Geometry check sheet. Reference: the model listing, model coordinates, mm. Face numbers are marked on the shaded views. A direction names the side the tool comes from. Give positions to 0.01 mm unless a question says otherwise; leave off trailing zeros. Loops run counter-clockwise (first coordinate to the right, second up) from the corner with the lowest first, then second, coordinate; pieces in that order, holes last. Notation, with made-up numbers: (-15.5, 73.5) - (1.5, 73.5) arc R20 ccw to (1.5, 103.5) - close; hole circle Ø10 at (-26.75, 29). An arc over 180 degrees is marked (long way). Use a Markdown table: item, result. Add a question column.
1. Depth check by flat-ended pin: P1, Ø4.5, axis at x = 20, z = 20, coming from the +Y side. Enter the tip coordinate at first touch or a pass-through.
2. Material ranges on L1, parallel to X at y = 4.5, z = 20; L2, parallel to X at y = 2, z = -20 (3 decimals), recorded low to high.
3. Cross-section at C-C on x = 0. Enter the section's corners in (y, z) (3 decimals).
4. Cross-section at B-B on y = 1.5. Enter the section's corners in (x, z) (3 decimals), and give its area (3 significant figures).
5. Draft check along X on the marked faces 1, 2 and 3. Enter one of: pulls with the +X half, pulls with the -X half, needs draft (parallel to the pull), parting line crosses it, or undercut.
6. Cross-section at D-D on y = 7.25. Enter the section's corners in (x, z) (3 decimals), and give its area (3 significant figures).
7. Set-up check for the marked faces 4 and 5: record each of +Z, -Z, +X, -X, +Y, -Y from which the full face is reachable in a straight line by a thin tool's end or side.
8. Cross-section at A-A on z = -1. Enter the section's corners in (x, y) (3 decimals), and give its area (3 significant figures).
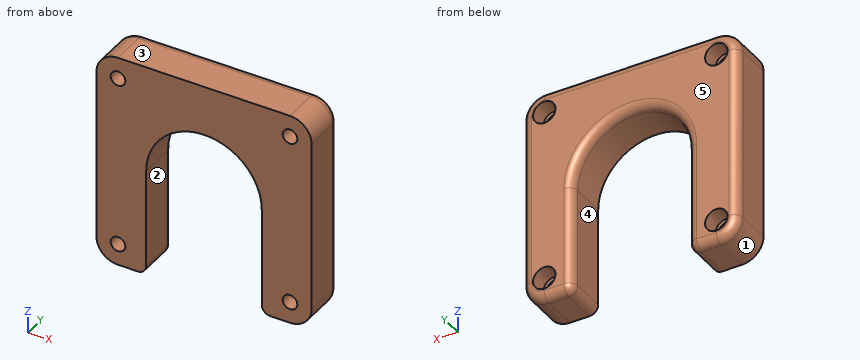
from build123d import *

# Parameters (mm, degrees)
BOSS_EXTRUDE1_DEPTH          = 10
SKETCH1_4_R                  = 1.7
CUT_EXTRUDE1_DEPTH           = 37.742346142
CUT_EXTRUDE2_START           = 10
SKETCH1_5_R                  = 2.6
CUT_EXTRUDE2_DEPTH           = 3.9
CUT_EXTRUDE2_DRAFT           = -1.5
CUT_EXTRUDE2_PROFILE_2_DEPTH = 3.9
CUT_EXTRUDE2_PROFILE_2_DRAFT = -1.5
CUT_EXTRUDE2_PROFILE_3_DEPTH = 3.9
CUT_EXTRUDE2_PROFILE_3_DRAFT = -1.5
CUT_EXTRUDE2_PROFILE_4_DEPTH = 3.9
CUT_EXTRUDE2_PROFILE_4_DRAFT = -1.5
FILLET1_R                    = 2
FILLET2_R                    = 2


with BuildPart() as part:
    # Sketch1 → Boss-Extrude1 (new body)
    with BuildSketch(Plane(origin=(0, 0, 0), x_dir=(1, 0, 0), z_dir=(0, 1, 0))):
        with BuildLine():
            Line((-20, -25), (20, -25))
            ThreePointArc((20, -25), (23.535533906, -23.535533906), (25, -20))
            Line((25, -20), (25, 20))
            ThreePointArc((25, 20), (23.535533906, 23.535533906), (20, 25))
            Line((20, 25), (-20, 25))
            ThreePointArc((-20, 25), (-23.535533906, 23.535533906), (-25, 20))
            Line((-25, 20), (-25, -20))
            ThreePointArc((-25, -20), (-23.535533906, -23.535533906), (-20, -25))
        make_face()
    extrude(amount=BOSS_EXTRUDE1_DEPTH)

    # Sketch1<4> → Cut-Extrude1 (cut, through all)
    with BuildSketch(Plane(origin=(0, 0, 0), x_dir=(1, 0, 0), z_dir=(0, 1, 0))):
        with BuildLine():
            Line((13.435, 25), (-13.435, 25))
            Line((-13.435, 25), (-13.435, 0))
            ThreePointArc((-13.435, 0), (0, -13.435), (13.435, 0))
            Line((13.435, 0), (13.435, 25))
        make_face()
        with Locations(Location((-20, 20, 0), (0, 0, 270))):
            Circle(SKETCH1_4_R)
        with Locations(Location((-20, -20, 0), (0, 0, 90))):
            Circle(SKETCH1_4_R)
        with Locations(Location((20, -20, 0), (0, 0, 90))):
            Circle(SKETCH1_4_R)
        with Locations(Location((20, 20, 0), (0, 0, 270))):
            Circle(SKETCH1_4_R)
    extrude(amount=CUT_EXTRUDE1_DEPTH, mode=Mode.SUBTRACT)


with BuildPart() as cut_extrude2_tool:
    # Sketch1<5> → Cut-Extrude2 (with draft: the straight prism first)
    with BuildSketch(Plane(origin=(0, 0, 0), x_dir=(1, 0, 0), z_dir=(0, 1, 0)).offset(CUT_EXTRUDE2_START)):
        with Locations((-20, 20)):
            Circle(SKETCH1_5_R)
    extrude(amount=-CUT_EXTRUDE2_DEPTH)
    # Cut-Extrude2: the draft: its side faces are tilted about the plane it starts from
    cut_extrude2_sides = [cut_extrude2_tool.faces().sort_by_distance(p)[0] for p in [
        (-22.6, 8.05, -20),
    ]]
    draft(cut_extrude2_sides, Plane(origin=(0, 0, 0), x_dir=(1, 0, 0), z_dir=(0, 1, 0)).offset(CUT_EXTRUDE2_START), CUT_EXTRUDE2_DRAFT)


with BuildPart() as part_1:
    add(part.part)

    # Cut-Extrude2: cut by cut_extrude2_tool
    add(cut_extrude2_tool.part, mode=Mode.SUBTRACT)


with BuildPart() as cut_extrude2_profile_2_tool:
    # Sketch1<5> → Cut-Extrude2 profile 2 (with draft: the straight prism first)
    with BuildSketch(Plane(origin=(0, 0, 0), x_dir=(1, 0, 0), z_dir=(0, 1, 0)).offset(CUT_EXTRUDE2_START)):
        with Locations((20, 20)):
            Circle(SKETCH1_5_R)
    extrude(amount=-CUT_EXTRUDE2_PROFILE_2_DEPTH)
    # Cut-Extrude2 profile 2: the draft: its side faces are tilted about the plane it starts from
    cut_extrude2_profile_2_sides = [cut_extrude2_profile_2_tool.faces().sort_by_distance(p)[0] for p in [
        (17.4, 8.05, -20),
    ]]
    draft(cut_extrude2_profile_2_sides, Plane(origin=(0, 0, 0), x_dir=(1, 0, 0), z_dir=(0, 1, 0)).offset(CUT_EXTRUDE2_START), CUT_EXTRUDE2_PROFILE_2_DRAFT)


with BuildPart() as part_2:
    add(part_1.part)

    # Cut-Extrude2 profile 2: cut by cut_extrude2_profile_2_tool
    add(cut_extrude2_profile_2_tool.part, mode=Mode.SUBTRACT)


with BuildPart() as cut_extrude2_profile_3_tool:
    # Sketch1<5> → Cut-Extrude2 profile 3 (with draft: the straight prism first)
    with BuildSketch(Plane(origin=(0, 0, 0), x_dir=(1, 0, 0), z_dir=(0, 1, 0)).offset(CUT_EXTRUDE2_START)):
        with Locations((-20, -20)):
            Circle(SKETCH1_5_R)
    extrude(amount=-CUT_EXTRUDE2_PROFILE_3_DEPTH)
    # Cut-Extrude2 profile 3: the draft: its side faces are tilted about the plane it starts from
    cut_extrude2_profile_3_sides = [cut_extrude2_profile_3_tool.faces().sort_by_distance(p)[0] for p in [
        (-22.6, 8.05, 20),
    ]]
    draft(cut_extrude2_profile_3_sides, Plane(origin=(0, 0, 0), x_dir=(1, 0, 0), z_dir=(0, 1, 0)).offset(CUT_EXTRUDE2_START), CUT_EXTRUDE2_PROFILE_3_DRAFT)


with BuildPart() as part_3:
    add(part_2.part)

    # Cut-Extrude2 profile 3: cut by cut_extrude2_profile_3_tool
    add(cut_extrude2_profile_3_tool.part, mode=Mode.SUBTRACT)


with BuildPart() as cut_extrude2_profile_4_tool:
    # Sketch1<5> → Cut-Extrude2 profile 4 (with draft: the straight prism first)
    with BuildSketch(Plane(origin=(0, 0, 0), x_dir=(1, 0, 0), z_dir=(0, 1, 0)).offset(CUT_EXTRUDE2_START)):
        with Locations((20, -20)):
            Circle(SKETCH1_5_R)
    extrude(amount=-CUT_EXTRUDE2_PROFILE_4_DEPTH)
    # Cut-Extrude2 profile 4: the draft: its side faces are tilted about the plane it starts from
    cut_extrude2_profile_4_sides = [cut_extrude2_profile_4_tool.faces().sort_by_distance(p)[0] for p in [
        (17.4, 8.05, 20),
    ]]
    draft(cut_extrude2_profile_4_sides, Plane(origin=(0, 0, 0), x_dir=(1, 0, 0), z_dir=(0, 1, 0)).offset(CUT_EXTRUDE2_START), CUT_EXTRUDE2_PROFILE_4_DRAFT)


with BuildPart() as part_4:
    add(part_3.part)

    # Cut-Extrude2 profile 4: cut by cut_extrude2_profile_4_tool
    add(cut_extrude2_profile_4_tool.part, mode=Mode.SUBTRACT)

    # Fillet1
    fillet1_edges = [part_4.edges().sort_by_distance(p)[0] for p in [
        (-13.435, 10, -12.5),
        (-13.435, 5, -25),
        (13.435, 5, -25),
        (0, 10, 13.435),
        (13.435, 10, -12.5),
    ]]
    fillet(fillet1_edges, radius=FILLET1_R)

    # Fillet2
    # the kernel refuses this fillet: 2 mm, written as the material it takes off along each edge
    with BuildSketch(Plane(origin=(15.435, 8, -23), x_dir=(0, 1, 0), z_dir=(0, 0, -1))) as fillet2_piece_1_section:
        Polygon((0, 0), (FILLET2_R, 0), (FILLET2_R, -FILLET2_R), (0, -FILLET2_R), align=None)
    fillet2_piece_1 = extrude(amount=FILLET2_R, mode=Mode.PRIVATE)
    fillet2_piece_1 = fillet2_piece_1 - Plane(origin=(15.435, 8, -23), x_dir=(0.7071067811865475, -0.7071067811865475, 0), z_dir=(0, 0, -1)) * Sphere(FILLET2_R, mode=Mode.PRIVATE)
    add(fillet2_piece_1, mode=Mode.SUBTRACT)
    with BuildSketch(Plane(origin=(-15.435, 8, -23), x_dir=(0, 1, 0), z_dir=(0, 0, -1))) as fillet2_piece_2_section:
        Polygon((0, 0), (FILLET2_R, 0), (FILLET2_R, FILLET2_R), (0, FILLET2_R), align=None)
    fillet2_piece_2 = extrude(amount=FILLET2_R, mode=Mode.PRIVATE)
    fillet2_piece_2 = fillet2_piece_2 - Plane(origin=(-15.435, 8, -23), x_dir=(-0.7071067811865475, -0.7071067811865475, 0), z_dir=(0, 0, -1)) * Sphere(FILLET2_R, mode=Mode.PRIVATE)
    add(fillet2_piece_2, mode=Mode.SUBTRACT)
    with BuildSketch(Plane(origin=(-20, 10, -20), x_dir=(0, 0, -1), z_dir=(1, 0, 0))) as fillet2_piece_3:
        with BuildLine():
            CenterArc((5 - FILLET2_R, -FILLET2_R), FILLET2_R, 0, 90)
            Line((5 - FILLET2_R, 0), (5, 0))
            Line((5, 0), (5, -FILLET2_R))
        make_face()
    revolve(axis=Axis((-20, 10, -20), (0, 1, 0)), revolution_arc=90, mode=Mode.SUBTRACT)
    with BuildSketch(Plane(origin=(-15.435, 10, -25), x_dir=(0, -1, 0), z_dir=(-1, 0, 0)), Plane(origin=(20, 10, -25), x_dir=(0, -1, 0), z_dir=(-1, 0, 0))) as fillet2_piece_4:
        with BuildLine():
            CenterArc((FILLET2_R, FILLET2_R), FILLET2_R, 180, 90)
            Line((0, FILLET2_R), (0, 0))
            Line((0, 0), (FILLET2_R, 0))
        make_face()
    extrude(amount=4.565, mode=Mode.SUBTRACT)
    with BuildSketch(Plane(origin=(20, 10, -20), x_dir=(1, 0, 0), z_dir=(0, 0, 1))) as fillet2_piece_5:
        with BuildLine():
            CenterArc((5 - FILLET2_R, -FILLET2_R), FILLET2_R, 0, 90)
            Line((5 - FILLET2_R, 0), (5, 0))
            Line((5, 0), (5, -FILLET2_R))
        make_face()
    revolve(axis=Axis((20, 10, -20), (0, 1, 0)), revolution_arc=90, mode=Mode.SUBTRACT)
    with BuildSketch(Plane(origin=(25, 10, 20), x_dir=(0, -1, 0), z_dir=(0, 0, -1)), Plane(origin=(-20, 10, 25), x_dir=(0, -1, 0), z_dir=(1, 0, 0)), Plane(origin=(-25, 10, -20), x_dir=(0, -1, 0), z_dir=(0, 0, 1))) as fillet2_piece_6:
        with BuildLine():
            CenterArc((FILLET2_R, FILLET2_R), FILLET2_R, 180, 90)
            Line((0, FILLET2_R), (0, 0))
            Line((0, 0), (FILLET2_R, 0))
        make_face()
    extrude(amount=40, mode=Mode.SUBTRACT)
    with BuildSketch(Plane(origin=(20, 10, 20), x_dir=(0, 0, 1), z_dir=(-1, 0, 0))) as fillet2_piece_7:
        with BuildLine():
            CenterArc((5 - FILLET2_R, -FILLET2_R), FILLET2_R, 0, 90)
            Line((5 - FILLET2_R, 0), (5, 0))
            Line((5, 0), (5, -FILLET2_R))
        make_face()
    revolve(axis=Axis((20, 10, 20), (0, 1, 0)), revolution_arc=90, mode=Mode.SUBTRACT)
    with BuildSketch(Plane(origin=(-20, 10, 20), x_dir=(-1, 0, 0), z_dir=(0, 0, -1))) as fillet2_piece_8:
        with BuildLine():
            CenterArc((5 - FILLET2_R, -FILLET2_R), FILLET2_R, 0, 90)
            Line((5 - FILLET2_R, 0), (5, 0))
            Line((5, 0), (5, -FILLET2_R))
        make_face()
    revolve(axis=Axis((-20, 10, 20), (0, 1, 0)), revolution_arc=90, mode=Mode.SUBTRACT)


solid = part_4.part
Values found:
| question | item | result |
|---|---|---|
| 1 | P1 | stops at y = 6.1 |
| 2 | L1 | x = -25 to -21.7, -18.3 to 18.3, 21.7 to 25 |
| 2 | L2 | x = -25 to -21.7, -18.3 to -13.435, 13.435 to 18.3, 21.7 to 25 |
| 3 | outline | (0, 13.435) - (8, 13.435) arc R2 ccw to (10, 15.435) - (10, 23) arc R2 ccw to (8, 25) - (0, 25) - close |
| 4 | outline | (-25, -20) arc R5 ccw to (-20, -25) - (-15.435, -25) arc R2 ccw to (-13.435, -23) - (-13.435, 0) arc R13.435 cw to (13.435, 0) - (13.435, -23) arc R2 ccw to (15.435, -25) - (20, -25) arc R5 ccw to (25, -20) - (25, 20) arc R5 ccw to (20, 25) - (-20, 25) arc R5 ccw to (-25, 20) - close; hole circle Ø3.4 at (-20, -20); hole circle Ø3.4 at (-20, 20); hole circle Ø3.4 at (20, -20); hole circle Ø3.4 at (20, 20) |
| 4 | area | 1,490 mm2 |
| 5 | face 1 | pulls with the -X half |
| 5 | face 2 | undercut |
| 5 | face 3 | needs draft |
| 6 | outline | (-25, -20) arc R5 ccw to (-20, -25) - (-15.435, -25) arc R2 ccw to (-13.435, -23) - (-13.435, 0) arc R13.435 cw to (13.435, 0) - (13.435, -23) arc R2 ccw to (15.435, -25) - (20, -25) arc R5 ccw to (25, -20) - (25, 20) arc R5 ccw to (20, 25) - (-20, 25) arc R5 ccw to (-25, 20) - close; hole circle Ø5.056 at (-20, -20); hole circle Ø5.056 at (-20, 20); hole circle Ø5.056 at (20, -20); hole circle Ø5.056 at (20, 20) |
| 6 | area | 1,440 mm2 |
| 7 | face 4 | -Z, +Y, -Y |
| 7 | face 5 | +Z, -Z, +X, -X, +Y |
| 8 | outline | (-25, 0) - (-13.435, 0) - (-13.435, 8) arc R2 ccw to (-15.435, 10) - (-23, 10) arc R2 ccw to (-25, 8) - close; (13.435, 0) - (25, 0) - (25, 8) arc R2 ccw to (23, 10) - (15.435, 10) arc R2 ccw to (13.435, 8) - close |
| 8 | area | 228 mm2 |
